```python
from build123d import *

# Parameters (mm, degrees)
F1_DEPTH = 200
F4_D     = 3
F6_D     = 5


with BuildPart() as f1:
    # F0 (on Front) → F1 (new body)
    with BuildSketch(Plane.XZ):
        Polygon((-11.212291, -34.163514), (14.787709, -34.163514), (14.787709, -30.163514), (-15.212291, -30.163514), (-15.212291, -60.163514), (-11.212291, -60.163514), align=None)
    extrude(amount=-F1_DEPTH)

    # F4 (through all)
    with Locations(Plane(origin=(-15.212291, 0, 0), x_dir=(0, -1, 0), z_dir=(-1, 0, 0))):
        with Locations((-20, -45.163514), (-80, -45.163514), (-180, -45.163514)):
            Hole(F4_D / 2)

    # F6 (through all)
    with Locations(Plane.XY.offset(-30.163514)):
        with Locations((-0.212291, 185), (-0.212291, 15)):
            Hole(F6_D / 2)


solid = f1.part
```
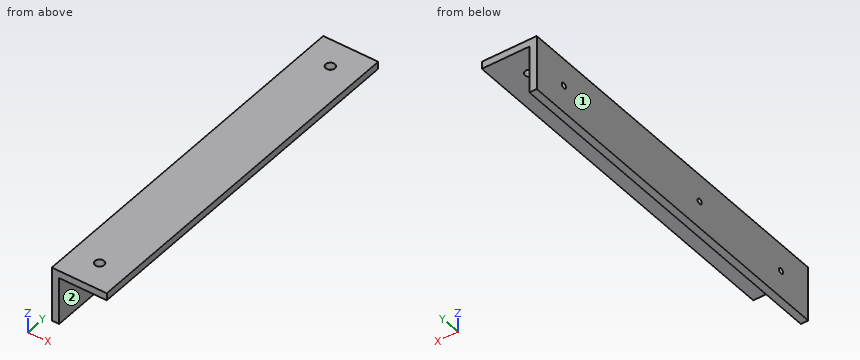
Geometry check sheet. Reference: the model listing, model coordinates, mm. Face numbers are marked on the shaded views. A direction names the side the tool comes from. Coordinates: 2 decimals unless noted, no trailing zeros. Order: outer loops, then holes, each group sorted by start corner. A loop starts at its lowest first (then second) coordinate and runs counter-clockwise, first axis right, second up.
Item 1: Tool access check on the marked faces 1 and 2. Record the directions out of +Z, -Z, +X, -X, +Y, -Y that give a thin tool (end or side, any length) a straight path to the whole face; none if there is none.
Item 2: Section check C-C (x = 6.25). Enter the section's corners in (y, z), plus the area to 3 significant figures.
Item 3: Depth check by flat-ended pin: pin 1 (4 mm diameter, centred on y = 70, z = -49, fed in from +X); pin 2 (1.8 mm diameter, centred on y = 20, z = -45.16, fed in from -X); pin 3 (8 mm diameter, centred on x = 10.5, y = 107, fed in from -Z). Enter the tip coordinate at first touch or a pass-through.
Item 4: Section check A-A (y = 185). Enter the section's corners in (x, z).
Item 5: Scan lines: line 1 along X through (y, z) = (185, -32.4); line 2 along Z through (x, y) = (-12.45, 80); line 3 along X through (y, z) = (157.5, -47). Record each from-to range of solid material in increasing order.
Item 6: Section check B-B (z = -42). Enter the section's corners in (x, y), plus the area to 3 significant figures.
Check sheet entries:
1. face 1: +Z, -Z, -X, +Y, -Y
1. face 2: -Z, +X, +Y, -Y
2. outline: (0, -34.16) - (200, -34.16) - (200, -30.16) - (0, -30.16) - close
2. area: 800 mm2
3. pin 1: stops at x = -11.21
3. pin 2: passes through
3. pin 3: stops at z = -34.16
4. outline: (-15.21, -60.16) - (-11.21, -60.16) - (-11.21, -34.16) - (-2.71, -34.16) - (-2.71, -30.16) - (-15.21, -30.16) - close; (2.29, -34.16) - (14.79, -34.16) - (14.79, -30.16) - (2.29, -30.16) - close
5. line 1: x = -15.21 to -2.71, 2.29 to 14.79
5. line 2: z = -60.16 to -46.66, -43.66 to -30.16
5. line 3: x = -15.21 to -11.21
6. outline: (-15.21, 0) - (-11.21, 0) - (-11.21, 200) - (-15.21, 200) - close
6. area: 800 mm2
